Autodesk Inventor part; units mm, degrees
ref_plane "YZ Plane" through (0, 0, 0) normal (1, 0, 0) x (0, 1, 0)
ref_plane "XZ Plane" through (0, 0, 0) normal (0, 1, 0) x (-1, 0, 0)
ref_plane "XY Plane" through (0, 0, 0) normal (0, 0, 1) x (1, 0, 0)
sketch "Sketch1" plane through (0, 0, 0) normal (0, 0, 1) x (1, 0, 0)
  line L0 (0, 0) -> (3.175, 0)
  line L1 (3.175, 0) -> (3.175, 12.7)
  line L2 (3.175, 12.7) -> (0, 12.7)
  line L3 (0, 12.7) -> (0, 0)
  line L4 (84.963, 0) -> (88.138, 0)
  line L5 (88.138, 0) -> (88.138, 12.7)
  line L6 (88.138, 12.7) -> (84.963, 12.7)
  line L7 (84.963, 12.7) -> (84.963, 0)
  arc A0 (84.963, 12.7) -> (3.175, 12.7) centre (44.069, -94.3642) ccw
  line L8 (0, 12.7) -> (0, 15.2331)
  line L9 (88.138, 12.7) -> (88.138, 15.2331)
  arc A1 (88.138, 15.2331) -> (0, 15.2331) centre (44.069, -94.3642) ccw
  dimension "d0" = 3.175
  dimension "d1" = 12.7
  dimension "d2" = 81.788
  dimension "d3" = 3.175
  dimension "d4" = 12.7
  dimension "d5" = 2.5331
  dimension "d6" = 2.5331
extrude "Extrusion1" add sketch "Sketch1" along normal blind 85.09
equation "\"d3\" = d0"
equation "\"d4\" = d1"
equation "\"d6\" = d5"
properties part number "Canopy"
For this review, take the finished solid that the model builds, in its own axes (mm). A direction names the side the tool comes from. Give positions to 0.01 mm unless a question says otherwise; leave off trailing zeros. Write each loop counter-clockwise with the first axis right and the second up, starting at its lowest first coordinate (ties: lowest second). Pieces come first, ordered by that corner, then holes. Notation, with made-up numbers: M 83.25,26 L 120.25,26 A32 cw 120.25,65 Z; hole C 7.5,-19.75 d8. An arc over 180 degrees is marked long. One line per item, written item: value.
1) For line 1 (X direction, y = 11, z = 12.5) (3 decimals); line 2 (Y direction, x = 45.5, z = 41); line 3 (Y direction, x = 54.5, z = 18), list the stretches that pass through material, from the lowest coordinate up. Write a range as from..to.
Results are:
line 1: x = 0..3.175, 84.963..88.138
line 2: y = 20.24..23.75
line 3: y = 19.77..23.3
2) Take a section at D-D, the plane x = 58.5. Write out the cut boundary in (y, z), then the cut area to 3 significant figures.
Results are:
outline: M 19.33,0 L 22.88,0 L 22.88,85.09 L 19.33,85.09 Z
area: 302 mm²
3) Take a section at A-A, the plane y = 2.25. Write out the cut boundary in (x, z) (3 decimals).
Results are:
outline: M 0,0 L 3.175,0 L 3.175,85.09 L 0,85.09 Z; M 84.963,0 L 88.138,0 L 88.138,85.09 L 84.963,85.09 Z
4) For P1, Ø10, axis at y = 2.5, z = 47, coming from the -X side; P2, Ø1, axis at x = 27, z = 11.5, coming from the -Y side; P3, Ø1, axis at x = 20, z = 60, coming from the -Y side; P4, Ø10, axis at x = 68, z = 20, coming from the +Y side, all flat-tipped, find the tip position at first contact; note any pin that passes through.
Results are:
P1: stops at x = 0
P2: stops at y = 18.89
P3: stops at y = 17.58
P4: stops at y = 22.23
5) Take a section at B-B, the plane z = 40.5. Write out the cut boundary in (x, y) (3 decimals).
Results are:
outline: M 0,0 L 3.175,0 L 3.175,12.7 A114.608 cw 84.963,12.7 L 84.963,0 L 88.138,0 L 88.138,15.233 A118.126 ccw 0,15.233 Z
6) The part is to be moulded in two halves that separate along X. For faces 3 (the flat face through (0, 8, 42)), 4 (the flat face through (3.175, 6, 42)), 5 (the flat face through (88.138, 8, 42)), 6 (the flat face through (41, 21, 85.09)), say which applies: +X half, -X half, draft (parallel to the pull), parting line (faces both ways), or undercut.
Results are:
face 3: -X half
face 4: undercut
face 5: +X half
face 6: draft
7) For faces 1 (the flat face through (84.963, 6, 42)), 2 (the flat face through (87, 0, 42)), list the 3-axis set-ups (+Z, -Z, +X, -X, +Y, -Y) from which the entire face can be reached by the end or side of a thin tool; tool diameter is ignored.
Results are:
face 1: +Z, -Z, -Y
face 2: +Z, -Z, +X, -X, -Y
8) Take a section at C-C, the plane y = 13.75. Write out the cut boundary in (x, z), then the cut area to 3 significant figures.
Results are:
outline: M 0,0 L 6.04,0 L 6.04,85.09 L 0,85.09 Z; M 82.1,0 L 88.14,0 L 88.14,85.09 L 82.1,85.09 Z
area: 1,030 mm²
